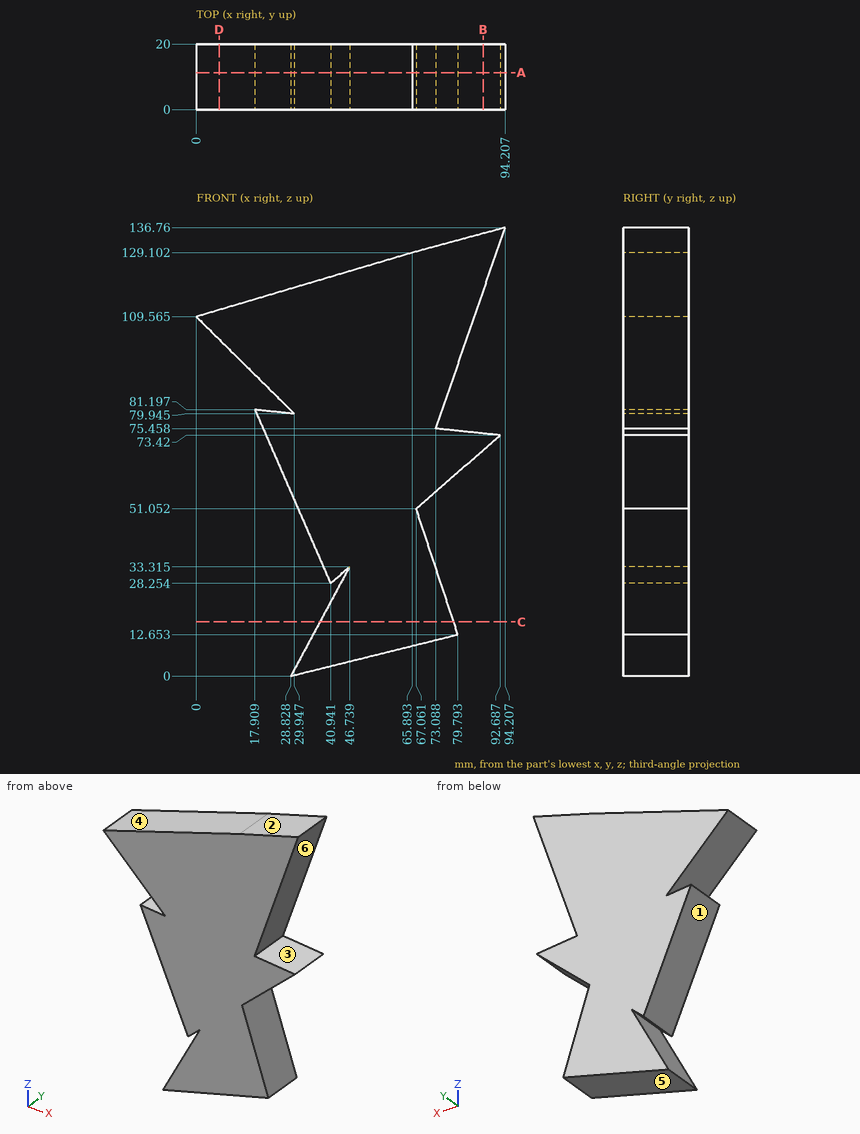
Part print with two shaded views. Sizes in mm from the minimum x, y, z corner. A direction names the side the tool comes from. Coordinates: 2 decimals unless noted, no trailing zeros. Write each loop counter-clockwise with the first axis right and the second up, starting at its lowest first coordinate (ties: lowest second). Pieces come first, ordered by that corner, then holes.
(1) Drill centre lines: line 1 (Z direction, x = 63, y = 19.25) (1 decimal); line 2 (X direction, y = 6, z = 86) (1 decimal); line 3 (Z direction, x = 64, y = 12.75). Where is each one in solid material? Low to high.
(2) 3-axis set-ups, long thin cutter, end or side, ignore diameter. For the marked faces 1, 2 and 3: which of +Z, -Z, +X, -X, +Y, -Y reach the whole face in a straight line?
(3) Pin check, flat tips, straight feed: pin 1 Ø12 at (y, z) = (9, 98.5) entering from -X; pin 2 Ø1 at (x, y) = (55.5, 10) entering from +Z; pin 3 Ø2 at (x, y) = (21, 3.5) entering from -Z (1 decimal). Stop position of each tip, or through.
(4) Mould opens along Z. For the marked faces 4, 5 and 6 say: pulls with the +Z half, pulls with the -Z half, needs draft (parallel to the pull), parting line crosses it, or undercut.
(5) Cut at C-C on z = 16.5. List the corners of the cut face in (x, y).
(6) Cut at B-B on x = 87.5. List the corners of the cut face in (y, z).
(7) Cut at D-D on x = 7. List the corners of the cut face in (y, z).
(8) Cut at A-A on y = 11.25. List the corners of the cut face in (x, z) (1 decimal), and give its area (4 significant figures).
Working result:
1. line 1: z = 8.5 to 128.2
1. line 2: x = 23.8 to 76.7
1. line 3: z = 8.73 to 128.54
2. face 1: -X, +Y, -Y
2. face 2: +Z, -X, +Y, -Y
2. face 3: +X, +Y, -Y
3. pin 1: stops at x = 5.12
3. pin 2: stops at z = 126.17
3. pin 3: stops at z = 71.8
4. face 4: pulls with the +Z half
4. face 5: pulls with the -Z half
4. face 6: undercut
5. outline: (37.7, 0) - (78.52, 0) - (78.52, 20) - (37.7, 20) - close
6. outline: (0, 68.89) - (20, 68.89) - (20, 73.96) - (0, 73.96) - close; (0, 117.29) - (20, 117.29) - (20, 134.95) - (0, 134.95) - close
7. outline: (0, 102.64) - (20, 102.64) - (20, 111.64) - (0, 111.64) - close
8. outline: (0, 109.6) - (29.9, 79.9) - (17.9, 81.2) - (40.9, 28.3) - (46.7, 33.3) - (28.8, 0) - (79.8, 12.7) - (67.1, 51.1) - (92.7, 73.4) - (73.1, 75.5) - (94.2, 136.8) - (65.9, 129.1) - close
8. area: 6,325 mm2
